Here's how the part is built. I have some questions about the finished solid (model axes, mm). A direction names the side the tool comes from. Round coordinates to 2 decimals unless told otherwise and drop trailing zeros. Loops run counter-clockwise (first coordinate to the right, second up) from the corner with the lowest first, then second, coordinate; pieces in that order, holes last. Notation, with made-up numbers: M -17.75,-8 L 30.25,-8 A24 cw 30.25,4 Z; hole C 88.5,-8 d5. An arc over 180 degrees is marked long. Write each question's results on one line, items separated by ' | '. Start each with the question number.
```python
from build123d import *

# Parameters (mm, degrees)
EXTRUDE_1_DEPTH     = 2
SKETCH_2_R          = 1.55
CUT_EXTRUDE_1_DEPTH = 22.950475716
SKETCH_3_R          = 1.05
CUT_EXTRUDE_2_DEPTH = 22.950475716
FILLET_2_R          = 3
EXTRUDE_2_DEPTH     = 2
FILLET_4_R          = 3


with BuildPart() as part:
    # 草图1 → 凸台-拉伸1 (new body)
    with BuildSketch(Plane(origin=(0, 0, 0), x_dir=(1, 0, 0), z_dir=(0, 1, 0))):
        Polygon((-19.437679495, -10), (19.437679495, -10), (15, 10), (-15, 10), align=None)
    extrude(amount=EXTRUDE_1_DEPTH)

    # 草图2 → 切除-拉伸1 (cut, through all)
    with BuildSketch(Plane(origin=(0, 2, 0), x_dir=(1, 0, 0), z_dir=(0, 1, 0))):
        with Locations(Location((-13.01801017, 5, 0), (0, 0, 270))):
            Circle(SKETCH_2_R)
        with Locations(Location((-13.01801017, -5, 0), (0, 0, 270))):
            Circle(SKETCH_2_R)
        with Locations(Location((13.01801017, -5, 0), (0, 0, 90))):
            Circle(SKETCH_2_R)
        with Locations(Location((13.01801017, 5, 0), (0, 0, 90))):
            Circle(SKETCH_2_R)
    extrude(amount=-CUT_EXTRUDE_1_DEPTH, mode=Mode.SUBTRACT)

    # 草图3 → 切除-拉伸2 (cut, through all)
    with BuildSketch(Plane(origin=(0, 2, 0), x_dir=(1, 0, 0), z_dir=(0, 1, 0))):
        with Locations(Location((-7.5, 8.5, 0), (0, 0, 270))):
            Circle(SKETCH_3_R)
        with Locations(Location((-7.5, -6.5, 0), (0, 0, 270))):
            Circle(SKETCH_3_R)
        with Locations(Location((7.5, -6.5, 0), (0, 0, 270))):
            Circle(SKETCH_3_R)
        with Locations(Location((7.5, 8.5, 0), (0, 0, 270))):
            Circle(SKETCH_3_R)
    extrude(amount=-CUT_EXTRUDE_2_DEPTH, mode=Mode.SUBTRACT)

    # 圆角2
    fillet_2_edges = [part.edges().sort_by_distance(p)[0] for p in [
        (-15, 1, -10),
        (15, 1, -10),
        (19.437679495, 1, 10),
        (-19.437679495, 1, 10),
    ]]
    fillet(fillet_2_edges, radius=FILLET_2_R)

    # 草图4 → 凸台-拉伸2 (add)
    with BuildSketch(Plane(origin=(0, 2, 0), x_dir=(1, 0, 0), z_dir=(0, 1, 0))):
        with BuildLine():
            ThreePointArc((-4.901923789, 10), (-7.5, 11.5), (-10.098076211, 10))
            Line((-10.098076211, 10), (-4.901923789, 10))
        make_face()
        with BuildLine():
            ThreePointArc((10.098076211, 10), (7.5, 11.5), (4.901923789, 10))
            Line((4.901923789, 10), (10.098076211, 10))
        make_face()
    extrude(amount=-EXTRUDE_2_DEPTH)

    # 圆角4
    fillet_4_edges = [part.edges().sort_by_distance(p)[0] for p in [
        (10.098076211, 1, -10),
        (4.901923789, 1, -10),
        (-4.901923789, 1, -10),
        (-10.098076211, 1, -10),
    ]]
    fillet(fillet_4_edges, radius=FILLET_4_R)


solid = part.part
```
1. I want a section at C-C on y = 0.65. Count the separate pieces of the cut face and the enclosed holes in it, plus the area to 3 significant figures.
2. I want a section at B-B on z = -8.5. List the corners of the cut face in (x, y) for me.
3. Which directions (+Z, -Z, +X, -X, +Y, -Y) give clear straight access to the entire face, cutting with the end or side of a thin tool? Please do faces 4 (the face through (-12, 1, -10)), 5 (the face through (12, 1, -10)), 6 (the face through (-14, 1, -6.2)), 7 (the face through (0, 1, -10)).
4. I want a section at A-A on x = 7.5. List the corners of the cut face in (y, z) for me.
5. For pin 1 (0.9 mm diameter, centred on x = -12, y = 1.5, fed in from -Z), with a flat end and sliding along its axis, tell me the tip position at first contact or that it passes through.
6. I want a section at D-D on x = 0. List the corners of the cut face in (y, z) for me.
7. If we mould it in two halves opening along Z, with no side actions, what happens to faces 1 (the face through (14.492, 1.014, -9.322)), 2 (the face through (0, 2, 1)), 3 (the face through (7.82, 1.01, -7.5))? For each: released by +Z, released by -Z, zero draft, split by the parting line, or undercut.
8. I need wall thicknesses on line 1 along X through (y, z) = (1.45, -5); line 2 along X through (y, z) = (0.4, -9.25); line 3 along Z through (x, y) = (3, 1.95). Which ranges of each line are inside material? Lowest first, please.
Outcome:
1) separate pieces: 1 | enclosed holes: 8 | area: 648 mm2
2) outline: M -15.19,0 L -8.55,0 L -8.55,2 L -15.19,2 Z; M -6.45,0 L 6.45,0 L 6.45,2 L -6.45,2 Z; M 8.55,0 L 15.19,0 L 15.19,2 L 8.55,2 Z
3) face 4: -Z, -X, +Y, -Y | face 5: -Z, +X, +Y, -Y | face 6: +Y, -Y | face 7: -Z, +Y, -Y
4) outline: M 0,-11.5 L 2,-11.5 L 2,-9.55 L 0,-9.55 Z; M 0,-7.45 L 2,-7.45 L 2,5.45 L 0,5.45 Z; M 0,7.55 L 2,7.55 L 2,10 L 0,10 Z
5) pin 1: z = -10
6) outline: M 0,-10 L 2,-10 L 2,10 L 0,10 Z
7) face 1: released by -Z | face 2: zero draft | face 3: undercut
8) line 1: -16.11 to -14.57, -11.47 to 11.47, 14.57 to 16.11 | line 2: -14.58 to -8.23, -6.77 to 6.77, 8.23 to 14.58 | line 3: -10 to 10
